```python
from build123d import *

# Parameters (mm, degrees)
F0_R     = 50
F1_DEPTH = 20
F2_R     = 25
F3_DEPTH = 7
F4_R     = 7
F5_DEPTH = 50.001
F6_R     = 7
F7_DEPTH = 20


with BuildPart() as f1:
    # F0 (on Top) → F1 (new body)
    with BuildSketch(Plane.XY):
        Circle(F0_R)
    extrude(amount=F1_DEPTH)

    # F2 (on face) → F3 (cut)
    with BuildSketch(Plane.XY.offset(20)):
        Circle(F2_R)
    extrude(amount=-F3_DEPTH, mode=Mode.SUBTRACT)

    # F4 (on Right) → F5 (cut, through all)
    with BuildSketch(Plane.YZ):
        with Locations((0, 20)):
            Circle(F4_R)
    extrude(amount=F5_DEPTH, mode=Mode.SUBTRACT)

    # F6 (on face) → F7 (cut)
    with BuildSketch(Plane.XY.offset(13)):
        with Locations((0, 13)):
            Circle(F6_R)
        with Locations((0, -13)):
            Circle(F6_R)
    extrude(amount=-F7_DEPTH, mode=Mode.SUBTRACT)


solid = f1.part
```
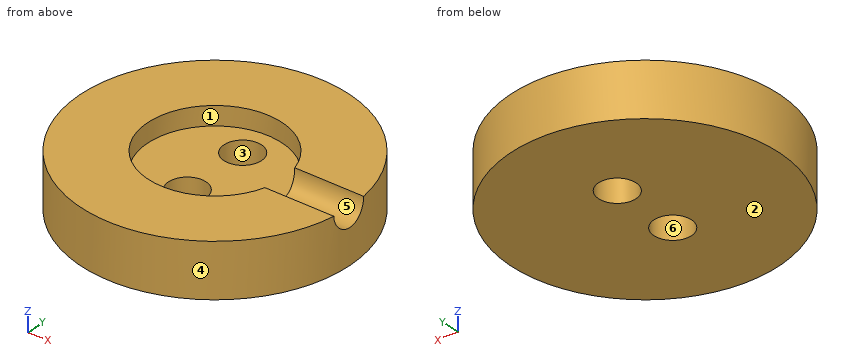
Geometry: final body of the model. Coordinates: model frame, mm. Face numbers are marked on the shaded views. A direction names the side the tool comes from. Give positions to 0.01 mm unless a question says otherwise; leave off trailing zeros. Order: outer loops, then holes, each group sorted by start corner. A loop starts at its lowest first (then second) coordinate and runs counter-clockwise, first axis right, second up. Notation, with made-up numbers: (83.25, 75) -> (124.25, 75) arc R13 cw to (124.25, 95) -> close; hole circle Ø2 at (86.5, 59). An arc over 180 degrees is marked (long way). Write each question's results on one line, items separated by ' | '. Start each with the question number.
1) Section A-A (x = 0). Return loops of the section in (y, z).
2) Section C-C (z = 1.5). Return loops of the section in (x, y).
3) Line query: line 1 (Y direction, x = 0, z = 7.5); line 2 (Y direction, x = -1, z = 1.75); line 3 (Y direction, x = 0, z = 17.25). Output: solid intervals per line, ascending. Write a range as from..to.
4) Set-up query: the marked faces 1 and 2. Return all of +Z, -Z, +X, -X, +Y, -Y with unobstructed straight access to the full face (end or side cutting, diameter ignored); none if empty.
5) Draft query along X for the marked faces 3, 4, 5 and 6. Return one class per face: pulls with the +X half, pulls with the -X half, needs draft (parallel to the pull), parting line crosses it, or undercut.
6) First-contact query: pin 1 (2 mm diameter, centred on x = 1, y = -18.5, fed in from -Z); pin 2 (6 mm diameter, centred on y = 36, z = 2, fed in from -X); pin 3 (22.5 mm diameter, centred on x = 0, y = -13, fed in from +Z); pin 4 (6 mm diameter, centred on x = -23, z = 6, fed in from +Y). Flat tips, straight axial feed; report the tip coordinate or a pass-through.
7) Section D-D (x = 20). Return loops of the section in (y, z).
8) Section B-B (y = 13). Return loops of the section in (x, z), then the cut area to 3 significant figures.
Calculated:
1) outline: (-50, 0) -> (-20, 0) -> (-20, 13) -> (-25, 13) -> (-25, 20) -> (-50, 20) -> close; (-6, 0) -> (6, 0) -> (6, 13) -> (-6, 13) -> close; (20, 0) -> (50, 0) -> (50, 20) -> (25, 20) -> (25, 13) -> (20, 13) -> close
2) outline: circle Ø100 at (0, 0); hole circle Ø14 at (0, -13); hole circle Ø14 at (0, 13)
3) line 1: -50..-20, -6..6, 20..50 | line 2: -49.99..-19.93, -6.07..6.07, 19.93..49.99 | line 3: -50..-25, 25..50
4) face 1: +Z | face 2: -Z, +X, -X, +Y, -Y
5) face 3: undercut | face 4: parting line crosses it | face 5: needs draft | face 6: undercut
6) pin 1: through | pin 2: x = -37.56 | pin 3: z = 13 | pin 4: y = 45.83
7) outline: (-45.83, 0) -> (45.83, 0) -> (45.83, 20) -> (15, 20) -> (15, 13) -> (-15, 13) -> (-15, 20) -> (-45.83, 20) -> close
8) outline: (-48.28, 0) -> (-7, 0) -> (-7, 13) -> (-21.35, 13) -> (-21.35, 20) -> (-48.28, 20) -> close; (7, 0) -> (48.28, 0) -> (48.28, 20) -> (21.35, 20) -> (21.35, 13) -> (7, 13) -> close | area: 1,450 mm2
